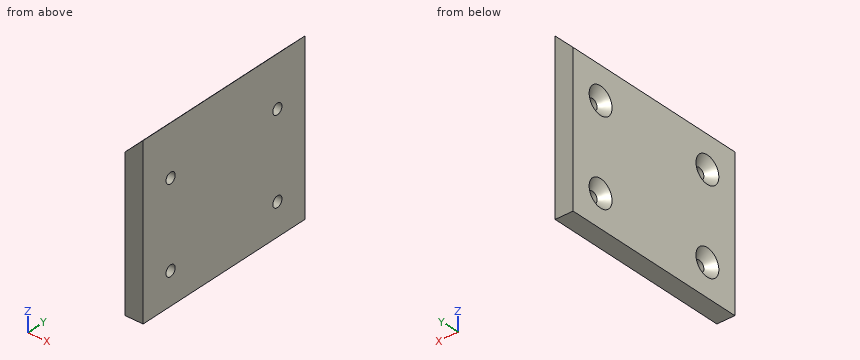
from build123d import *

# Parameters (mm, degrees)
F1_DEPTH       = 53
F3_D           = 3
F3_CSINK_D     = 7.5
F3_CSINK_ANGLE = 90


with BuildPart() as f1:
    # F0 (on Front) → F1 (new body)
    with BuildSketch(Plane.XZ):
        Polygon((0, 41.5), (0, 0), (5, 0), (5, 46.5), align=None)
    extrude(amount=F1_DEPTH)

    # F3 (through all)
    with Locations(Plane(origin=(0, 0, 0), x_dir=(0, -1, 0), z_dir=(-1, 0, 0))):
        with Locations((9, 32.5), (44, 32.5), (44, 9), (9, 9)):
            CounterSinkHole(F3_D / 2, F3_CSINK_D / 2, counter_sink_angle=F3_CSINK_ANGLE)


solid = f1.part
Could you check a few things on this model? Use its own coordinates, in mm. Round coordinates to 2 decimals unless told otherwise and drop trailing zeros. Write each loop counter-clockwise with the first axis right and the second up, starting at its lowest first coordinate (ties: lowest second). Pieces come first, ordered by that corner, then holes. Notation, with made-up numbers: (48, 34.5) -> (64, 34.5) arc R36 ccw to (64, 72.5) -> close; hole circle Ø6 at (-38.75, 27). An arc over 180 degrees is marked (long way). Use a Markdown table: item, result.
1. Please list where these lines run through material, in increasing order: probe 1 along Y at (x, z) = (4.1, 32.5); probe 2 along Z at (x, y) = (3.8, -9); probe 3 along Z at (x, y) = (3.6, -44).
Answer key:
| item | result |
|---|---|
| probe 1 | y = -53 to -45.5, -42.5 to -10.5, -7.5 to 0 |
| probe 2 | z = 0 to 7.5, 10.5 to 31, 34 to 45.3 |
| probe 3 | z = 0 to 7.5, 10.5 to 31, 34 to 45.1 |
2. If we section it at D-D (y = -26): List the corners of the cut face in (x, z) for me, then the cut area to 3 significant figures.
Answer key:
| item | result |
|---|---|
| outline | (0, 0) -> (5, 0) -> (5, 46.5) -> (0, 41.5) -> close |
| area | 220 mm^2 |
3. For pin 1 Ø3.5 at (y, z) = (-44, 9) entering from -X; pin 2 Ø1 at (y, z) = (-7.5, 38) entering from -X; pin 3 Ø1.5 at (x, y) = (2.5, -25.5) entering from +Z, each with a flat end and sliding along its axis, tell me the tip position at first contact or that it passes through.
Answer key:
| item | result |
|---|---|
| pin 1 | stops at x = 2 |
| pin 2 | stops at x = 0 |
| pin 3 | stops at z = 44.75 |
4. If we section it at C-C (y = -44): List the corners of the cut face in (x, z) for me.
Answer key:
| item | result |
|---|---|
| outline | (0, 0) -> (5, 0) -> (5, 7.5) -> (2.25, 7.5) -> (0, 5.25) -> close; (0, 12.75) -> (2.25, 10.5) -> (5, 10.5) -> (5, 31) -> (2.25, 31) -> (0, 28.75) -> close; (0, 36.25) -> (2.25, 34) -> (5, 34) -> (5, 46.5) -> (0, 41.5) -> close |
5. If we section it at B-B (x = 0.95): List the corners of the cut face in (y, z) for me, then the cut area to 3 significant figures.
Answer key:
| item | result |
|---|---|
| outline | (-53, 0) -> (0, 0) -> (0, 42.45) -> (-53, 42.45) -> close; hole circle Ø5.6 at (-44, 9); hole circle Ø5.6 at (-44, 32.5); hole circle Ø5.6 at (-9, 9); hole circle Ø5.6 at (-9, 32.5) |
| area | 2,150 mm^2 |
6. If we section it at A-A (z = 9): List the corners of the cut face in (x, y) for me.
Answer key:
| item | result |
|---|---|
| outline | (0, -53) -> (5, -53) -> (5, -45.5) -> (2.25, -45.5) -> (0, -47.75) -> close; (0, -40.25) -> (2.25, -42.5) -> (5, -42.5) -> (5, -10.5) -> (2.25, -10.5) -> (0, -12.75) -> close; (0, -5.25) -> (2.25, -7.5) -> (5, -7.5) -> (5, 0) -> (0, 0) -> close |
